Work out the finished part from the listing and answer in its coordinate system (mm). A direction names the side the tool comes from. Give positions to 0.01 mm unless a question says otherwise; leave off trailing zeros. Loops run counter-clockwise (first coordinate to the right, second up) from the corner with the lowest first, then second, coordinate; pieces in that order, holes last. Notation, with made-up numbers: (-40, -8.5) - (-6, -8.5) arc R12 ccw to (-6, 10.5) - close; hole circle Ø7 at (36.25, 69). An arc over 180 degrees is marked (long way). One line per question, with ' | ' between items. Start each with the question number.
1. Section C-C (z = 4.5) is taken. Determine the outline of the cut face in (x, y) (3 decimals), plus the area to 3 significant figures.
2. Section A-A (x = -12.5) is taken. Give the number of separate pieces and of enclosed holes in the cut face, plus the area to 3 significant figures.
3. For a pull along Z with two mould halves and no side action, classify faces 5 (the face through (0, 19, -19.142)), 6 (the face through (-25.4, -7, -8)), 7 (the face through (-0.36, -10.84, 0.46)) as released by +Z, released by -Z, zero draft, split by the parting line, or undercut.
4. Which of the six approach directions +Z, -Z, +X, -X, +Y, -Y give full straight-line access (tool end or side, diameter ignored) to faces 1 (the face through (-3.175, 23, 0)), 2 (the face through (6, 33, -12.792)), 3 (the face through (-11.77, 6.66, -16.01)), 4 (the face through (3.175, 23, 0))?
5. Section D-D (z = -9.5) is taken. Determine the outline of the cut face in (x, y) (3 decimals), plus the area to 3 significant figures.
6. Find the intervals of material crossed by line 1 (Y direction, x = -14.5, z = -14.5); line 2 (Y direction, x = 7, z = 6.5); line 3 (Z direction, x = -8, y = 57), in increasing order.
7. Each of these flat-tipped pins is pushed along its axis until it touches: pin 1 (8 mm diameter, centred on x = -12, y = 35.5, fed in from +Z); pin 2 (4.5 mm diameter, centred on x = 0, z = -9, fed in from +Y); pin 3 (4 mm diameter, centred on y = 46, z = -1.5, fed in from +X) (3 decimals). Where does it stop, or does it pass through?
8. Section B-B (y = -11) is taken. Determine the outline of the cut face in (x, z).
from build123d import *

# Parameters (mm, degrees)
F1_DEPTH      = 25.4
F1_DEPTH_BACK = 25.4
F4_DEPTH      = 3.175
F4_DEPTH_BACK = 3.175
F6_D          = 19.05
F8_D          = 6.35


with BuildPart() as f1:
    # F0 (on Right) → F1 (new body, two sides)
    with BuildSketch(Plane.YZ) as f1_sk:
        Polygon((-5.696102, 18.957503), (-31.096102, 18.957503), (-31.096102, -19.142497), (70.503898, -19.142497), (70.503898, -12.792497), (-5.696102, -12.792497), align=None)
    extrude(amount=F1_DEPTH)
    extrude(f1_sk.sketch, amount=-F1_DEPTH_BACK)

    # F3 (on Right) → F4 (join, two sides)
    with BuildSketch(Plane.YZ) as f4_sk:
        Polygon((-5.919815, -13.259767), (70.482805, -13.227087), (70.482805, -6.877087), (-5.919815, 18.714948), align=None)
    extrude(amount=F4_DEPTH)
    extrude(f4_sk.sketch, amount=-F4_DEPTH_BACK)

    # F6 (through all)
    with Locations(Plane.YZ.offset(25.4)):
        with Locations((-18.396102, 6.257503)):
            Hole(F6_D / 2)

    # F8 (through all)
    with Locations(Plane.XY.offset(-12.792497)):
        with Locations((-14.2875, 8.591398), (-14.2875, 59.391398), (14.2875, 8.591398), (14.2875, 59.391398)):
            Hole(F8_D / 2)


solid = f1.part
Conclusion:
1) outline: (-25.4, -31.096) - (25.4, -31.096) - (25.4, -27.758) - (-25.4, -27.758) - close; (-25.4, -9.035) - (25.4, -9.035) - (25.4, -5.696) - (3.175, -5.696) - (3.175, 36.518) - (-3.175, 36.518) - (-3.175, -5.696) - (-25.4, -5.696) - close | area: 607 mm²
2) separate pieces: 3 | enclosed holes: 1 | area: 1,100 mm²
3) face 5: released by -Z | face 6: zero draft | face 7: undercut
4) face 1: +Z, -X, +Y | face 2: +Z, +Y | face 3: +Z, -Z | face 4: +Z, +X, +Y
5) outline: (-25.4, -31.096) - (25.4, -31.096) - (25.4, -5.696) - (3.175, -5.696) - (3.175, 70.483) - (-3.175, 70.483) - (-3.175, -5.696) - (-25.4, -5.696) - close | area: 1,770 mm²
6) line 1: -31.1 to 5.42, 11.76 to 56.22, 62.56 to 70.5 | line 2: -31.1 to -27.92, -8.87 to -5.7 | line 3: -19.14 to -12.79
7) pin 1: z = -12.79 | pin 2: y = 70.48 | pin 3: x = 3.175
8) outline: (-25.4, -19.14) - (25.4, -19.14) - (25.4, 0.26) - (-25.4, 0.26) - close; (-25.4, 12.26) - (25.4, 12.26) - (25.4, 18.96) - (-25.4, 18.96) - close
